Autodesk Inventor part; units mm, degrees
ref_plane "YZ Plane" through (0, 0, 0) normal (1, 0, 0) x (0, 1, 0)
ref_plane "XZ Plane" through (0, 0, 0) normal (0, 1, 0) x (-1, 0, 0)
ref_plane "XY Plane" through (0, 0, 0) normal (0, 0, 1) x (1, 0, 0)
sketch "Sketch1" plane through (0, 0, 0) normal (0, 1, 0) x (-1, 0, 0)
  line L0 (0, 0) -> (-34, 0)
  line L1 (-34, 0) -> (-34, -83)
  line L2 (-34, -83) -> (0, -83)
  line L3 (0, -83) -> (0, 0)
  line L4 (-10, -40) -> (-24, -40)
  line L5 (-24, -40) -> (-24, -44)
  line L6 (-24, -44) -> (-10, -44)
  line L7 (-10, -44) -> (-10, -40)
  line L8 (-17, 0) -> (-17, -40) construction
  line L9 (-10, -44) -> (-14, -40) construction
  line L10 (-24, -44) -> (-20, -40) construction
  point P0 (-22, -42)
  point P1 (-12, -42)
  dimension "d0" = 34
  dimension "d1" = 83
  dimension "d2" = 14
  dimension "d3" = 4
  dimension "d4" = 43
  dimension "d12" = 45
extrude "Extrusion1" add sketch "Sketch1" along normal blind 2.6 contours L3 L2 L1 L0 | L7 L6 L5 L4
extrude "Extrusion2" add sketch "Sketch1" against normal blind 3.4 contours L7 L6 L5 L4
sketch "Sketch2" plane through (0, -3.4, 0) normal (0, -1, 0) x (1, 0, 0)
  point P0 (0, 0)
  point P1 (22, -42)
  point P2 (12, -42)
hole "Hole1" at (22, -3.4, -42) at (12, -3.4, -42) direction (0, 1, 0) diameter 3.5 depth 8
fillet "Fillet1" radius 2 4 edges at (24, -1.7, -40) (24, -1.7, -44) (10, -1.7, -40) (10, -1.7, -44)
chamfer "Chamfer1" distance 0.5 angle 45 16 edges at (34, 0, -41.5) (34, 1.3, 0) (17, 0, 0) (0, 0, -41.5) (17, 0, -83) (17, 2.6, -83) (0, 1.3, -83) (34, 1.3, -83) (0, 1.3, 0) (10.5856, 0, -40.5856) (17, 0, -44) (23.4144, 0, -40.5856) (17, 0, -40) (34, 2.6, -41.5) (17, 2.6, 0) (0, 2.6, -41.5)
properties part number "Game-Piece-Funnel-Pusher-Plate"
The listing builds one solid part. Answer for the finished solid, in the listing's coordinates (mm). A direction names the side the tool comes from. Round coordinates to 2 decimals unless told otherwise and drop trailing zeros. Write each loop counter-clockwise with the first axis right and the second up, starting at its lowest first coordinate (ties: lowest second). Pieces come first, ordered by that corner, then holes. Notation, with made-up numbers: M -27.75,57.5 L 27.25,57.5 A27 ccw 27.25,87.5 Z; hole C 67.5,70.25 d11. An arc over 180 degrees is marked long. Write each question's results on one line, items separated by ' | '. Start each with the question number.
(1) The part is cut by section B-B, the plane x = 25.5. Write down the section's boundary in (y, z).
(2) The part is cut by section A-A, the plane y = -1.65. Give the number of separate pieces and of enclosed holes in the cut face, and give its area (3 significant figures).
(3) For faces 1 (the cylindrical face through (10.57, -1.97, -43.4)), 2 (the cylindrical face through (23.4, -1.97, -43.43)), 3 (the cylindrical face through (23.43, -1.97, -40.6)), 4 (the flat face through (17, -2, -44)), 5 (the cylindrical face through (10.6, -1.97, -40.57)), determine the directions among +Z, -Z, +X, -X, +Y, -Y from which every point of the face is accessible in a straight line to the end or side of a thin tool.
(4) Each of these flat-tipped pins is pushed along its axis until it touches: P1, Ø1.4, axis at x = 15.5, y = -2.5, coming from the +Z side; P2, Ø2.5, axis at x = 16.5, y = -1.5, coming from the -Z side. Where does it stop, or does it pass through?
(5) The part is cut by section C-C, the plane z = -19. Write down the section's boundary in (x, y).
(6) Find the intervals of material crossed by line 1 (Z direction, x = 12, y = -1.5); line 2 (Y direction, x = 12.5, z = -57.5); line 3 (X direction, y = 0.35, z = -42), in increasing order.
(7) Determine the mould class of faces 6 (the cylindrical face through (11.474, -0.358, -43.669)), 7 (the cylindrical face through (20.5, -0.4, -42.9)), 8 (the flat face through (17, -2, -40)), 9 (the conical face through (10.5, -0.36, -43.53)) for opening direction Z: +Z half, -Z half, draft (parallel to the pull), parting line (faces both ways), or undercut.
Worked answers:
1) outline: M 0,-82.5 L 0.5,-83 L 2.1,-83 L 2.6,-82.5 L 2.6,-0.5 L 2.1,0 L 0.5,0 L 0,-0.5 Z
2) separate pieces: 1 | enclosed holes: 2 | area: 33.3 mm²
3) face 1: -Z, -X, -Y | face 2: -Z, +X, -Y | face 3: +Z, +X, -Y | face 4: -Z, +X, -X, -Y | face 5: +Z, -X, -Y
4) P1: stops at z = -40 | P2: stops at z = -44.25
5) outline: M 0,0.5 L 0.5,0 L 33.5,0 L 34,0.5 L 34,2.1 L 33.5,2.6 L 0.5,2.6 L 0,2.1 Z
6) line 1: z = -44 to -43.75, -40.25 to -40 | line 2: y = 0 to 2.6 | line 3: x = 0.15 to 10.25, 13.75 to 20.25, 23.75 to 33.85
7) face 6: undercut | face 7: undercut | face 8: +Z half | face 9: -Z half
